Could you check a few things on this model? Use its own coordinates, in mm. Face numbers are marked on the shaded views. A direction names the side the tool comes from. Give positions to 0.01 mm unless a question says otherwise; leave off trailing zeros. Loops run counter-clockwise (first coordinate to the right, second up) from the corner with the lowest first, then second, coordinate; pieces in that order, holes last.
1. Imagine slicing it at A-A (y = -1.5). List the corners of the cut face in (x, z) for me.
2. For P1, Ø5.5, axis at x = 1.5, y = 0, coming from the +Z side, with a flat end and sliding along its axis, tell me the tip position at first contact or that it passes through.
3. Imagine slicing it at C-C (z = 3.6). List the corners of the cut face in (x, y) for me.
4. I need wall thicknesses on line 1 along Y through (x, z) = (0, 1.2); line 2 along Y through (x, z) = (-2, 2.35). Which ranges of each line are inside material? Lowest first, please.
5. Thinking about a two-plate mould opening in X: for the marked faces 3, 4, 5 and 6, which applies, +X half, -X half, draft (parallel to the pull), parting line (faces both ways), or undercut?
6. For the marked faces 1 and 2, which set-ups out of +Z, -Z, +X, -X, +Y, -Y let a thin tool reach every point of the face, with its end or its side?
7. Imagine slicing it at D-D (y = 4.25). List the corners of the cut face in (x, z) for me, plus the area to 3 significant figures.
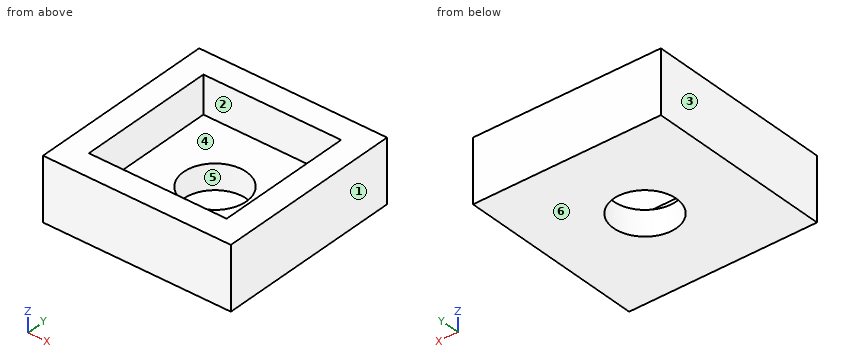
```python
from build123d import *

# Parameters (mm, degrees)
SKETCH_1_W          = 15
SKETCH_1_H          = 15
EXTRUDE_2_DEPTH     = 5
SHELL_1_T           = -2
SKETCH_2_R          = 2.5
CUT_EXTRUDE_1_DEPTH = 5


with BuildPart() as part:
    # 草图1 → 凸台-拉伸2 (new body)
    with BuildSketch(Plane.XY):
        Rectangle(SKETCH_1_W, SKETCH_1_H)
    extrude(amount=EXTRUDE_2_DEPTH)

    # 抽壳1
    shell_1_openings = [part.faces().sort_by_distance(p)[0] for p in [
        (0, 0, 5),
    ]]
    offset(amount=SHELL_1_T, openings=shell_1_openings, kind=Kind.INTERSECTION)

    # 草图2 → 切除-拉伸1 (cut)
    with BuildSketch(Plane(origin=(0, 0, 0), x_dir=(-1, 0, 0), z_dir=(0, 0, -1))):
        Circle(SKETCH_2_R)
    extrude(amount=-CUT_EXTRUDE_1_DEPTH, mode=Mode.SUBTRACT)


solid = part.part
```
Derived:
1. outline: (-7.5, 0) - (-2, 0) - (-2, 2) - (-5.5, 2) - (-5.5, 5) - (-7.5, 5) - close; (2, 0) - (7.5, 0) - (7.5, 5) - (5.5, 5) - (5.5, 2) - (2, 2) - close
2. P1: stops at z = 2
3. outline: (-7.5, -7.5) - (7.5, -7.5) - (7.5, 7.5) - (-7.5, 7.5) - close; hole (-5.5, -5.5) - (5.5, -5.5) - (5.5, 5.5) - (-5.5, 5.5) - close
4. line 1: y = -7.5 to -2.5, 2.5 to 7.5
4. line 2: y = -7.5 to -5.5, 5.5 to 7.5
5. face 3: -X half
5. face 4: undercut
5. face 5: undercut
5. face 6: draft
6. face 1: +Z, -Z, +X, +Y, -Y
6. face 2: +Z
7. outline: (-7.5, 0) - (7.5, 0) - (7.5, 5) - (5.5, 5) - (5.5, 2) - (-5.5, 2) - (-5.5, 5) - (-7.5, 5) - close
7. area: 42.0 mm2
